Part model, mm, in its own coordinate system. A direction names the side the tool comes from. Coordinates: 2 decimals unless noted, no trailing zeros. Order: outer loops, then holes, each group sorted by start corner. A loop starts at its lowest first (then second) coordinate and runs counter-clockwise, first axis right, second up.
1) Pin check, flat tips, straight feed: pin 1 Ø0.8 at (x, y) = (0, 8) entering from +Z; pin 2 Ø1.6 at (x, y) = (-8, 0) entering from +Z; pin 3 Ø1.2 at (x, y) = (11, -8) entering from +Z. Stop position of each tip, or through.
2) Cut at B-B (z = -11). Give the number of separate pieces and of enclosed holes in the cut face, and give its area (3 significant figures).
3) Cut at D-D (y = -32). List the corners of the cut face in (x, z), and give its area (3 significant figures).
4) Tool access for faces 4 (the cylindrical face through (9.667, -1.269, -35.014)), 5 (the cylindrical face through (5.495, -4.925, 1.014)), 6 (the cylindrical face through (0.2, -29.2, -11.62)): list every direction of +Z, -Z, +X, -X, +Y, -Y with a clear straight run to the whole face (end or side of a thin tool).
5) Mould opens along Y. For faces 1 (the flat face through (0, 11.25, -17)), 2 (the flat face through (14.25, -12, -17)), 3 (the cylindrical face through (11, -7, -17)) say: +Y half, -Y half, draft (parallel to the pull), parting line (faces both ways), or undercut.
6) Cut at C-C (z = -20.5). List the corners of the cut face in (x, y), and give its area (3 significant figures).
7) Wall check: L1, parallel to Y at x = 7, z = -23; L2, parallel to Y at x = 0, z = 0.95; L3, parallel to Y at x = -11, z = -24.5. Give the ranges that are in metal, low to high.
8) Cut at A-A (x = -11). List the corners of the cut face in (y, z).
Autodesk Inventor part; units mm, degrees
ref_plane "YZ Plane" through (0, 0, 0) normal (1, 0, 0) x (0, 1, 0)
ref_plane "XZ Plane" through (0, 0, 0) normal (0, 1, 0) x (-1, 0, 0)
ref_plane "XY Plane" through (0, 0, 0) normal (0, 0, 1) x (1, 0, 0)
sketch "Эскиз1" plane through (0, 0, 0) normal (0, 0, 1) x (1, 0, 0)
  line L0 (-12.25, 11.25) -> (12.25, 11.25)
  line L1 (14.25, 9.25) -> (14.25, -33.25)
  line L2 (12.25, -35.25) -> (-12.25, -35.25)
  line L3 (-14.25, -33.25) -> (-14.25, 9.25)
  circle A0 centre (-11, 8) radius 1
  circle A1 centre (-11, -8) radius 1
  circle A2 centre (11, 8) radius 1
  circle A3 centre (11, -8) radius 1
  circle A4 centre (11, -32) radius 1
  circle A5 centre (-11, -32) radius 1
  line L4 (-12.25, 11.25) -> (-14.25, 9.25)
  line L5 (12.25, 11.25) -> (14.25, 9.25)
  line L6 (14.25, -33.25) -> (12.25, -35.25)
  line L7 (-12.25, -35.25) -> (-14.25, -33.25)
  point P0 (0, 0)
  point P1 (-14.25, 11.25)
  point P2 (14.25, -35.25)
  point P3 (14.25, 11.25)
  point P4 (-14.25, -35.25)
  point P5 (0, 11.25)
  dimension "d0" = 28.5
  dimension "d1" = 46.5
  dimension "d2" = 11.25
  dimension "d3" = 22
  dimension "d4" = 11
  dimension "d5" = 8
  dimension "d6" = 8
  dimension "d7" = 40
  dimension "d8" = 2
  dimension "d11" = 2
  dimension "d12" = 2
  dimension "d13" = 2
  dimension "d14" = 2
  dimension "d15" = 2
  dimension "d16" = 2
  dimension "d17" = 2
  dimension "d18" = 2
extrude "Выдавливание1" add sketch "Эскиз1" against normal blind 34
sketch "Эскиз2" plane through (0, 0, 0) normal (1, 0, 0) x (0, 1, 0)
  line L0 (0, 0) -> (0, 7.2)
  line L1 (0, 7.2) -> (2.4047, 7.2)
  line L2 (2.4047, 7.2) -> (2.4047, 4.2)
  line L3 (2.4047, 4.2) -> (4, 4.2)
  line L4 (4, 4.2) -> (4, 2)
  line L5 (4, 2) -> (9.75, 2)
  line L6 (9.75, 2) -> (9.75, 0)
  line L7 (9.75, 0) -> (0, 0)
  line L8 (-33.25, -34) -> (9.25, -34)
  line L9 (0, -34) -> (9.75, -34)
  line L10 (9.75, -34) -> (9.75, -36)
  line L11 (9.75, -36) -> (0, -36)
  line L12 (0, -36) -> (0, -34)
  point P0 (1.2024, 7.2)
  dimension "d19" = 19.5
  dimension "d20" = 8
  dimension "d21" = 2
  dimension "d22" = 2.2
  dimension "d23" = 2
  dimension "d24" = 19.5
  dimension "d25" = 41.2
revolve "Вращение1" add sketch "Эскиз2" angle 360 about axis through (0, 0, 0) along (0, 0, 1)
sketch "Эскиз3" plane through (14.25, -33.25, 0) normal (1, 0, 0) x (0, 0, -1)
  circle A0 centre (11, 29.25) radius 1.35
  circle A1 centre (11, 5.25) radius 1.35
  circle A2 centre (23, 29.25) radius 1.35
  circle A3 centre (23, 5.25) radius 1.35
  line L0 (0, 0) -> (0, 42.5)
  line L1 (-7.2, 35.6547) -> (-7.2, 30.8453)
  line L2 (-7.2, 33.25) -> (42.1725, 33.25)
  point P0 (0, 33.25)
  dimension "d27" = 11
  dimension "d28" = 12
  dimension "d29" = 24
  dimension "d30" = 4
  dimension "d31" = 2.7
extrude "Выдавливание2" cut sketch "Эскиз3" against normal up to surface (28.5 mm away)
sketch "Эскиз4" plane through (0, 0, 2) normal (0, 0, 1) x (1, 0, 0)
  circle A0 centre (0, -8) radius 0.75
  point P0 (0, 0)
  dimension "d34" = 1.5
  dimension "d35" = 8
extrude "Выдавливание3" cut sketch "Эскиз4" against normal blind 2
pattern_circular "Круговой массив1" count 8 over 360 about axis through (0, 0, 1) along (0, 0, 1) of "Выдавливание3"
properties part number "DYNAMIXEL XM430-W350"
Geometry check:
1. pin 1: stops at z = 0
1. pin 2: stops at z = 2
1. pin 3: passes through
2. separate pieces: 3
2. enclosed holes: 6
2. area: 1,140 mm2
3. outline: (-14.25, -34) - (-12, -34) - (-12, 0) - (-14.25, 0) - close; (-10, -34) - (10, -34) - (10, 0) - (-10, 0) - close; (12, -34) - (14.25, -34) - (14.25, 0) - (12, 0) - close
3. area: 833 mm2
4. face 4: -Z
4. face 5: +Z
4. face 6: +X, -X
5. face 1: +Y half
5. face 2: draft
5. face 3: undercut
6. outline: (-14.25, -33.25) - (-12.25, -35.25) - (12.25, -35.25) - (14.25, -33.25) - (14.25, 9.25) - (12.25, 11.25) - (-12.25, 11.25) - (-14.25, 9.25) - close; hole circle Ø2 at (-11, -32); hole circle Ø2 at (-11, -8); hole circle Ø2 at (-11, 8); hole circle Ø2 at (11, -32); hole circle Ø2 at (11, -8); hole circle Ø2 at (11, 8)
6. area: 1,300 mm2
7. L1: y = -35.25 to -29.35, -26.65 to -5.35, -2.65 to 11.25
7. L2: y = -9.75 to -8.75, -7.25 to 7.25, 8.75 to 9.75
7. L3: y = -35.25 to -33, -31 to -9, -7 to 7, 9 to 11.25
8. outline: (-35.25, -34) - (-33, -34) - (-33, 0) - (-35.25, 0) - close; (-31, -34) - (-9, -34) - (-9, 0) - (-31, 0) - close; (-7, -34) - (7, -34) - (7, 0) - (-7, 0) - close; (9, -34) - (11.25, -34) - (11.25, 0) - (9, 0) - close; hole circle Ø2.7 at (-28, -23); hole circle Ø2.7 at (-28, -11); hole circle Ø2.7 at (-4, -23); hole circle Ø2.7 at (-4, -11)
